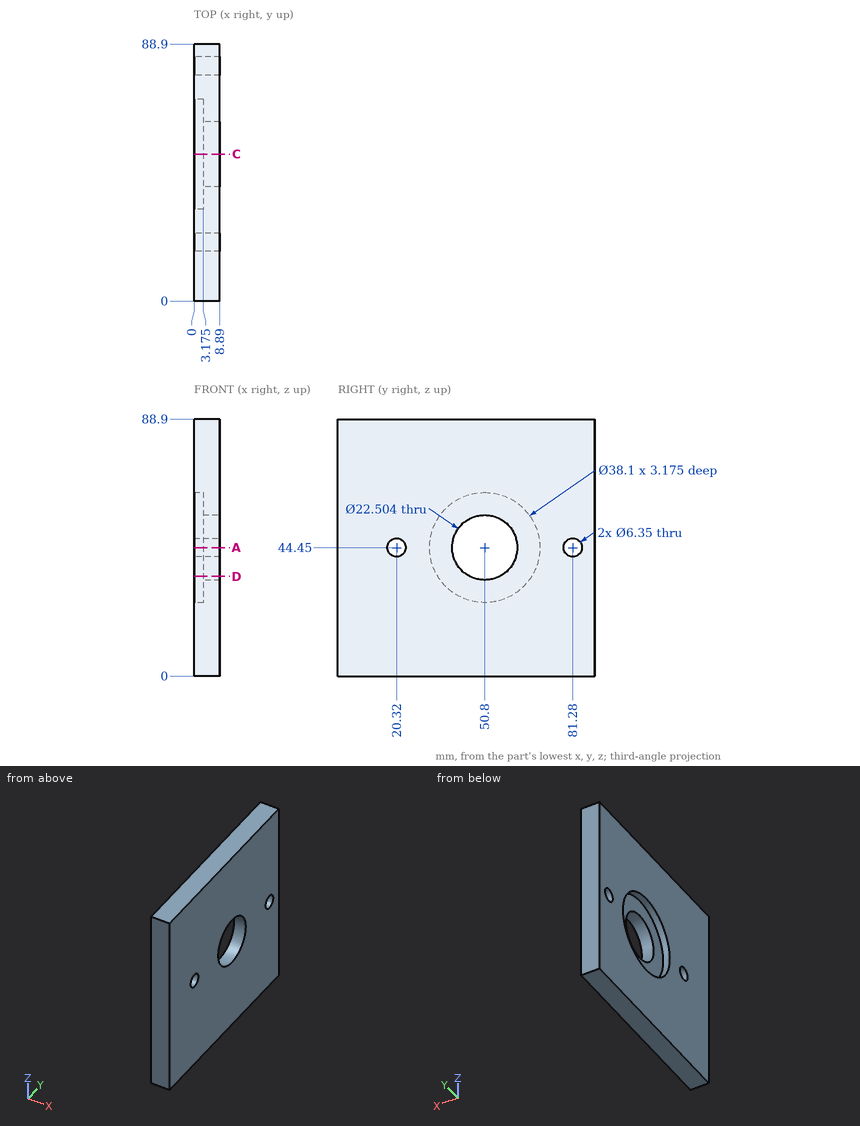
Drawing for the job (mm, zero at the part's lowest x, y, z). Give positions to 0.01 mm unless a question says otherwise; leave off trailing zeros. Write each loop counter-clockwise with the first axis right and the second up, starting at its lowest first coordinate (ties: lowest second). Pieces come first, ordered by that corner, then holes. Notation, with made-up numbers: M -11,22.5 L 2,22.5 A37 cw 2,58.5 Z; hole C 3,-18 d6. An arc over 180 degrees is marked long. Use CSV: the item, a comma, the result in double quotes.
Item 1: Drill centre lines: probe 1 along Z at (x, y) = (6.5, 40.5); probe 2 along Z at (x, y) = (4.75, 47.5); probe 3 along Y at (x, z) = (6, 54.5). Where is each one in solid material? Low to high.
Taken from the geometry:
probe 1,"z = 0 to 39.92, 48.98 to 88.9"
probe 2,"z = 0 to 33.69, 55.21 to 88.9"
probe 3,"y = 0 to 45.74, 55.86 to 88.9"
Item 2: Slice it at D-D on z = 34.5. Write the cut outline in (x, y) (1 decimal), plus the area to 3 significant figures.
Taken from the geometry:
outline,"M 0,0 L 8.9,0 L 8.9,45.5 L 3.2,45.5 L 3.2,34.6 L 0,34.6 Z; M 0,67 L 3.2,67 L 3.2,56.1 L 8.9,56.1 L 8.9,88.9 L 0,88.9 Z"
area,"627 mm²"
Item 3: Slice it at A-A on z = 44.45. State how many separate pieces and enclosed holes the cut face has, plus the area to 3 significant figures.
Taken from the geometry:
separate pieces,"4"
enclosed holes,"0"
area,"428 mm²"
Item 4: Slice it at C-C on y = 50.8. Write the cut outline in (x, z) (1 decimal).
Taken from the geometry:
outline,"M 0,0 L 8.9,0 L 8.9,33.2 L 3.2,33.2 L 3.2,25.4 L 0,25.4 Z; M 0,63.5 L 3.2,63.5 L 3.2,55.7 L 8.9,55.7 L 8.9,88.9 L 0,88.9 Z"
